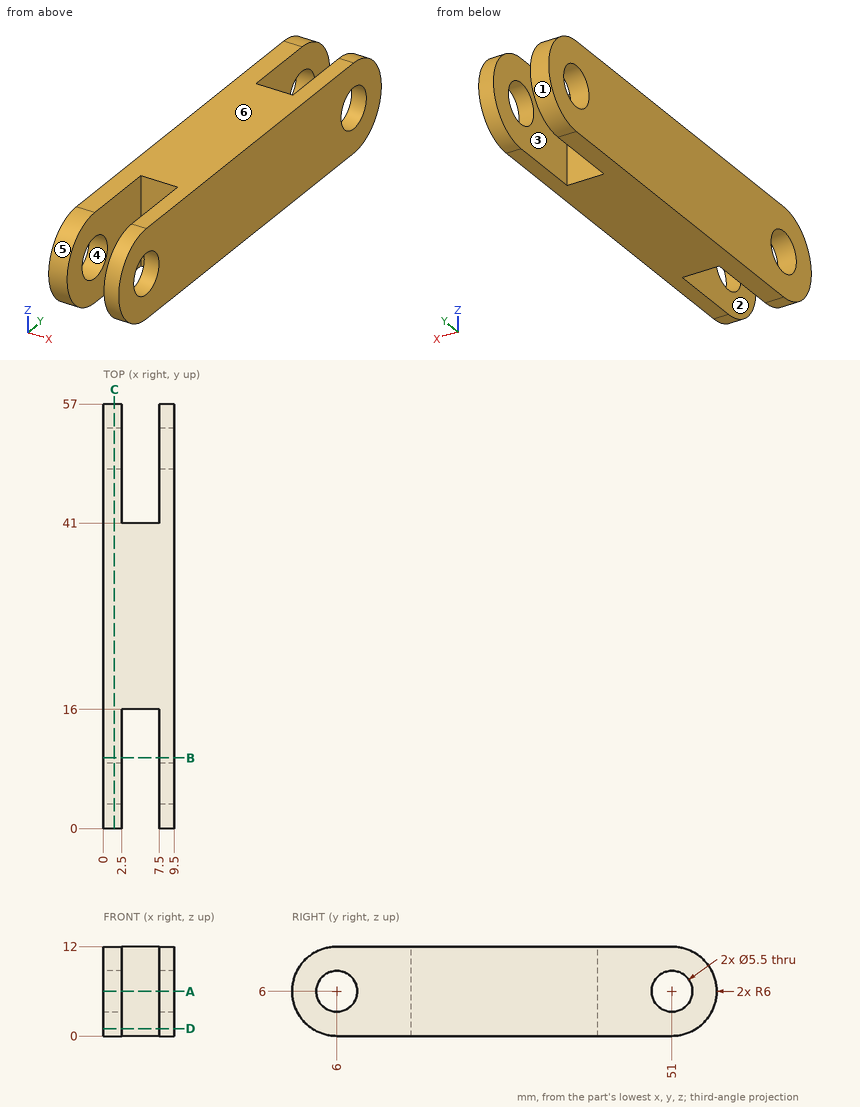
Answer from the drawing. Dimensions are ordinates in mm from the lowest x, y and z of the part. A direction names the side the tool comes from. Coordinates: 2 decimals unless noted, no trailing zeros. Order: outer loops, then holes, each group sorted by start corner. A loop starts at its lowest first (then second) coordinate and runs counter-clockwise, first axis right, second up. Notation, with made-up numbers: (-26.5, 77) - (-19.5, 77) arc R29 cw to (-19.5, 101) - close; hole circle Ø7 at (-32, 77.5). An arc over 180 degrees is marked (long way). Answer as a JSON object with one key per item and string values. Group by question number.
Item 1: Section B-B (y = 9.5) is taken. Give the vertices of the cut face in (x, z), plus the area to 3 significant figures.
Item 2: A tool of negligible diameter and unlimited length cuts with its end or side. For the marked faces 1, 2 and 3, from which of +Z, -Z, +X, -X, +Y, -Y can it reach the whole face along a straight path? Write none if from no direction.
Item 3: Flat-ended cylindrical pins translate along their axes: P1, Ø3.5, axis at y = 6, z = 6, coming from the -X side; P2, Ø4, axis at x = 6, z = 7.5, coming from the +Y side; P3, Ø3, axis at x = 1, z = 8, coming from the -Y side. Find the tip coordinate at first contact, or state that the pin passes through.
Item 4: Consider probe 1 along Y at (x, z) = (8.1, 6); probe 2 along Z at (x, y) = (1.6, 51); probe 3 along X at (y, z) = (45, 11.75). Determine where each line is inside the solid, lowest interval first. Write a range as from..to.
Item 5: The mould has two halves that part along Y. Classify the marked faces 4, 5 and 6: +Y half, -Y half, draft (parallel to the pull), parting line (faces both ways), or undercut.
Item 6: Section C-C (x = 1.5) is taken. Give the vertices of the cut face in (y, z), plus the area to 3 significant figures.
Item 7: Section A-A (z = 6) is taken. Give the vertices of the cut face in (x, y), plus the area to 3 significant figures.
Item 8: Section D-D (z = 1) is taken. Give the vertices of the cut face in (x, y).
Results are:
{
 "1": {"outline": "(0, 0) - (2.5, 0) - (2.5, 12) - (0, 12) - close; (7.5, 0) - (9.5, 0) - (9.5, 12) - (7.5, 12) - close", "area": "54.0 mm^2"},
 "2": {"face 1": "+X, -X, +Y", "face 2": "+Z, -Z, -Y", "face 3": "+Z, -Z, +Y"},
 "3": {"P1": "passes through", "P2": "stops at y = 57", "P3": "stops at y = 0.02"},
 "4": {"probe 1": "y = 0..3.25, 8.75..48.25, 53.75..57", "probe 2": "z = 0..3.25, 8.75..12", "probe 3": "x = 0..2.5, 7.5..9.5"},
 "5": {"face 4": "undercut", "face 5": "-Y half", "face 6": "draft"},
 "6": {"outline": "(6, 0) - (51, 0) arc R6 ccw to (51, 12) - (6, 12) arc R6 ccw to start; hole circle Ø5.5 at (6, 6); hole circle Ø5.5 at (51, 6)", "area": "606 mm^2"},
 "7": {"outline": "(0, 0) - (2.5, 0) - (2.5, 3.25) - (0, 3.25) - close; (0, 8.75) - (2.5, 8.75) - (2.5, 16) - (7.5, 16) - (7.5, 8.75) - (9.5, 8.75) - (9.5, 48.25) - (7.5, 48.25) - (7.5, 41) - (2.5, 41) - (2.5, 48.25) - (0, 48.25) - close; (0, 53.75) - (2.5, 53.75) - (2.5, 57) - (0, 57) - close; (7.5, 0) - (9.5, 0) - (9.5, 3.25) - (7.5, 3.25) - close; (7.5, 53.75) - (9.5, 53.75) - (9.5, 57) - (7.5, 57) - close", "area": "332 mm^2"},
 "8": {"outline": "(0, 2.68) - (2.5, 2.68) - (2.5, 16) - (7.5, 16) - (7.5, 2.68) - (9.5, 2.68) - (9.5, 54.32) - (7.5, 54.32) - (7.5, 41) - (2.5, 41) - (2.5, 54.32) - (0, 54.32) - close"}
}
